```python
from build123d import *

# Parameters (mm, degrees)
CYLINDER_R     = 2
CYLINDER_DEPTH = 10
BOX_W          = 10
BOX_H          = 10
BOX_DEPTH      = 3
ARRAY_X_COUNT  = 10
ARRAY_X_PITCH  = 10


with BuildPart() as cilindro:
    # Cylinder → Cylinder (new body)
    with BuildSketch(Plane(origin=(5, 5, -3), x_dir=(1, 0, 0), z_dir=(0, 0, 1))):
        Circle(CYLINDER_R)
    extrude(amount=CYLINDER_DEPTH)


with BuildPart() as obj1:
    # Box → Box (new body)
    with BuildSketch(Plane.XY):
        with Locations((5, 5)):
            Rectangle(BOX_W, BOX_H)
    extrude(amount=BOX_DEPTH)

    # Cut: cut Cilindro
    add(cilindro.part, mode=Mode.SUBTRACT)

    # Array X: obj1 ×10


with BuildPart() as obj1_1:
    add(obj1.part)
    with Locations(*[(i * ARRAY_X_PITCH, 0, 0) for i in range(1, ARRAY_X_COUNT)]):
        add(obj1.part)


solid = obj1_1.part
```
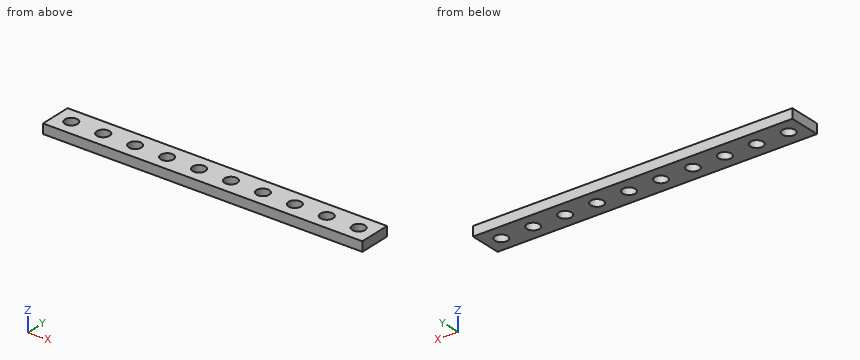
Here's how the part is built. I have some questions about the finished solid (model axes, mm). Coordinates: 2 decimals unless noted, no trailing zeros. Order: outer loops, then holes, each group sorted by start corner. A loop starts at its lowest first (then second) coordinate and runs counter-clockwise, first axis right, second up.
Item 1: If we section it at B-B, the plane x = 85: List the corners of the cut face in (y, z) for me.
Response values:
outline: (0, 0) - (3, 0) - (3, 3) - (0, 3) - close; (7, 0) - (10, 0) - (10, 3) - (7, 3) - close
Item 2: If we section it at D-D, the plane x = 35.5: List the corners of the cut face in (y, z) for me.
Response values:
outline: (0, 0) - (3.06, 0) - (3.06, 3) - (0, 3) - close; (6.94, 0) - (10, 0) - (10, 3) - (6.94, 3) - close
Item 3: I'm going to push flat-ended pins straight in: pin 1 Ø3 at (x, y) = (25, 5) entering from +Z; pin 2 Ø4.5 at (x, y) = (75, 5) entering from -Z. Where does each tip first touch, or does it pass through?
Response values:
pin 1: passes through
pin 2: stops at z = 0
Item 4: I need wall thicknesses on probe 1 along Y at (x, z) = (25, 1.3); probe 2 along Y at (x, z) = (25.5, 0.3). Which ranges of each line are inside material? Lowest first, please.
Response values:
probe 1: y = 0 to 3, 7 to 10
probe 2: y = 0 to 3.06, 6.94 to 10
Item 5: If we section it at A-A, the plane z = 1: Give the number of separate pieces and of enclosed holes in the cut face, then the cut area to 3 significant figures.
Response values:
separate pieces: 1
enclosed holes: 10
area: 874 mm2
